Source: CAD feature listing. Evaluate the final solid. Frame: model axes, mm. A direction names the side the tool comes from. Coordinates: 2 decimals unless noted, no trailing zeros. Order: outer loops, then holes, each group sorted by start corner. A loop starts at its lowest first (then second) coordinate and runs counter-clockwise, first axis right, second up. Notation, with made-up numbers: (-12.75, -3.75) -> (27.25, -3.75) arc R29 cw to (27.25, 32.25) -> close; hole circle Ø1 at (83.5, -31). An arc over 180 degrees is marked (long way). Write item = value, one per line. Start each with the question number.
Item 1: Ray query, line 1 along Y through (x, z) = (6, 0.9); line 2 along Y through (x, z) = (-2, 0.3); line 3 along X through (y, z) = (8, 0.9). Return the intervals inside material, ascending. Write a range as [from, to].
Item 2: Section query D-D (x = 8). Output: boundary loops of the cut face in (y, z), then the cut area to 3 significant figures.
Item 3: Contact query for flat-ended pins moving along their axis: pin 1 (0.8 mm diameter, centred on x = 4, z = 0.5, fed in from +Y); pin 2 (0.8 mm diameter, centred on x = -2.5, z = 0.5, fed in from -Y). Output: stop coordinate, or through.
Item 4: Section query B-B (x = -5). Output: boundary loops of the cut face in (y, z).
Item 5: Mould query, pull axis Y, two halves, no side actions, for faces 4 (the flat face through (14, 17, 1)), 5 (the flat face through (0, -11.75, 1)), 6 (the flat face through (-17, -17.75, 1)). Classes: released by +Y, released by -Y, zero draft, split by the parting line, or undercut.
Item 6: Section query A-A (y = 1.25). Output: boundary loops of the cut face in (x, z), then the cut area to 3 significant figures.
Item 7: Section query C-C (z = 0.6). Count the separate pieces of the cut face and the enclosed holes in it, then the cut area to 3 significant figures.
Item 8: Set-up query: faces 1 (the flat face through (17, 17.75, 1)), 2 (the flat face through (0, -13.75, 1)), 3 (the cylindrical face through (-6.53, -4.64, 0.74)). Return all of +Z, -Z, +X, -X, +Y, -Y with unobstructed straight access to the full face (end or side cutting, diameter ignored); none if empty.
```python
from build123d import *

# Parameters (mm, degrees)
F1_DEPTH = 1.5


# Not quite as in the source:
# - ends of sketch curves that miss each other by under 0.0002 mm in the source are joined


with BuildPart() as f1:
    # F0 (on Top) → F1 (new body)
    with BuildSketch(Plane.XY):
        with BuildLine():
            ThreePointArc((19.6082164698, -11.4503983868), (13.339608, 1.2499996959), (19.608215987, 13.9503980169))
            ThreePointArc((19.608215987, 13.9503980169), (19.8967236619, 14.3015730303), (20.000004, 14.744172))
            Line((20.000004, 14.744172), (20.000004, 17.25))
            ThreePointArc((20.000004, 17.25), (19.8535573906, 17.6035533906), (19.500004, 17.75))
            Line((19.500004, 17.75), (14.500004, 17.75))
            ThreePointArc((14.500004, 17.75), (14.1464506094, 17.6035533906), (14.000004, 17.25))
            Line((14.000004, 17.25), (14.000004, 16.25))
            ThreePointArc((14.000004, 16.25), (13.4441182966, 15.5255556337), (12.6004849604, 15.8749999771))
            ThreePointArc((12.6004849604, 15.8749999771), (12.3259659886, 16.1495190594), (11.950966, 16.25))
            Line((11.950966, 16.25), (-11.950958, 16.25))
            ThreePointArc((-11.950958, 16.25), (-12.3259579886, 16.1495190594), (-12.6004770396, 15.8750000229))
            ThreePointArc((-12.6004770396, 15.8750000229), (-13.4441102966, 15.5255556337), (-13.999996, 16.25))
            Line((-13.999996, 16.25), (-13.999996, 17.25))
            ThreePointArc((-13.999996, 17.25), (-14.1464426094, 17.6035533906), (-14.499996, 17.75))
            Line((-14.499996, 17.75), (-19.499996, 17.75))
            ThreePointArc((-19.499996, 17.75), (-19.8535493906, 17.6035533906), (-19.999996, 17.25))
            Line((-19.999996, 17.25), (-19.999996, 14.744172))
            ThreePointArc((-19.999996, 14.744172), (-19.8967156619, 14.3015730303), (-19.6082083041, 13.9503976031))
            ThreePointArc((-19.6082083041, 13.9503976031), (-13.3396, 1.2499996959), (-19.6082084698, -11.4503983868))
            ThreePointArc((-19.6082084698, -11.4503983868), (-19.8967227718, -11.8015703601), (-20.000004, -12.244173))
            Line((-20.000004, -12.244173), (-19.999996, -17.25))
            ThreePointArc((-19.999996, -17.25), (-19.8535493906, -17.6035533906), (-19.499996, -17.75))
            Line((-19.499996, -17.75), (-14.499996, -17.75))
            ThreePointArc((-14.499996, -17.75), (-14.1464426094, -17.6035533906), (-13.999996, -17.25))
            Line((-13.999996, -17.25), (-13.999996, -13.75))
            ThreePointArc((-13.999996, -13.75), (-13.4441102966, -13.0255556337), (-12.6004769604, -13.3749999771))
            ThreePointArc((-12.6004769604, -13.3749999771), (-12.3259579886, -13.6495190594), (-11.950958, -13.75))
            Line((-11.950958, -13.75), (11.950966, -13.75))
            ThreePointArc((11.950966, -13.75), (12.3259659886, -13.6495190594), (12.6004850396, -13.3750000229))
            ThreePointArc((12.6004850396, -13.3750000229), (13.4441182966, -13.0255556337), (14.000004, -13.75))
            Line((14.000004, -13.75), (14.000004, -17.25))
            ThreePointArc((14.000004, -17.25), (14.1464506094, -17.6035533906), (14.500004, -17.75))
            Line((14.500004, -17.75), (19.500004, -17.75))
            ThreePointArc((19.500004, -17.75), (19.8535573906, -17.6035533906), (20.000004, -17.25))
            Line((20.000004, -17.25), (20.000004, -12.244173))
            ThreePointArc((20.000004, -12.244173), (19.8967236619, -11.8015740303), (19.6082164698, -11.4503983868))
        make_face()
        with BuildLine():
            ThreePointArc((-8.6748168, -5.9830934), (-6.4973578405, -4.6318753463), (-3.9800720916, -5.1118651461))
            ThreePointArc((-3.9800720916, -5.1118651461), (3.5765e-06, -6.257042), (3.980079547, -5.1118658719))
            ThreePointArc((3.980079547, -5.1118658719), (6.4973651354, -4.631875401), (8.67482416, -5.98309388))
            Line((8.67482416, -5.98309388), (11.800004, -10.15))
            ThreePointArc((11.800004, -10.15), (11.894431191, -11.1972135955), (11.000004, -11.75))
            Line((11.000004, -11.75), (-10.999996, -11.75))
            ThreePointArc((-10.999996, -11.75), (-11.894423191, -11.1972135955), (-11.799996, -10.15))
            Line((-11.799996, -10.15), (-8.6748168, -5.9830934))
        make_face(mode=Mode.SUBTRACT)
        with BuildLine():
            ThreePointArc((9.000004, 2.95), (10.700004, 1.25), (9.000004, -0.45))
            Line((9.000004, -0.45), (-8.999996, -0.45))
            ThreePointArc((-8.999996, -0.45), (-10.699996, 1.25), (-8.999996, 2.95))
            Line((-8.999996, 2.95), (9.000004, 2.95))
        make_face(mode=Mode.SUBTRACT)
        with BuildLine():
            Line((-10.999996, 14.25), (11.000004, 14.25))
            ThreePointArc((11.000004, 14.25), (11.894431191, 13.6972135955), (11.800004, 12.65))
            Line((11.800004, 12.65), (8.674824, 8.483093))
            ThreePointArc((8.674824, 8.483093), (6.4973648742, 7.1318743525), (3.9800786415, 7.6118644285))
            ThreePointArc((3.9800786415, 7.6118644285), (3.5765e-06, 8.757041), (-3.9800718144, 7.6118647041))
            ThreePointArc((-3.9800718144, 7.6118647041), (-6.4973575792, 7.1318742978), (-8.6748168, 8.4830924))
            Line((-8.6748168, 8.4830924), (-11.799996, 12.65))
            ThreePointArc((-11.799996, 12.65), (-11.894423191, 13.6972135955), (-10.999996, 14.25))
        make_face(mode=Mode.SUBTRACT)
    extrude(amount=F1_DEPTH)


solid = f1.part
```
Computed:
q1.line_1 = [-13.75, -11.75], [-4.58, -0.45], [2.95, 7.08], [14.25, 16.25]
q1.line_2 = [-13.75, -11.75], [-5.99, -0.45], [2.95, 8.49], [14.25, 16.25]
q1.line_3 = [-14.83, -8.24], [-3.28, 3.28], [8.24, 14.83]
q2.outline = (-13.75, 0) -> (-11.75, 0) -> (-11.75, 1.5) -> (-13.75, 1.5) -> close; (-5.3, 0) -> (-0.45, 0) -> (-0.45, 1.5) -> (-5.3, 1.5) -> close; (2.95, 0) -> (7.8, 0) -> (7.8, 1.5) -> (2.95, 1.5) -> close; (14.25, 0) -> (16.25, 0) -> (16.25, 1.5) -> (14.25, 1.5) -> close
q2.area = 20.6 mm^2
q3.pin_1 = 16.25
q3.pin_2 = -13.75
q4.outline = (-13.75, 0) -> (-11.75, 0) -> (-11.75, 1.5) -> (-13.75, 1.5) -> close; (-4.68, 0) -> (-0.45, 0) -> (-0.45, 1.5) -> (-4.68, 1.5) -> close; (2.95, 0) -> (7.18, 0) -> (7.18, 1.5) -> (2.95, 1.5) -> close; (14.25, 0) -> (16.25, 0) -> (16.25, 1.5) -> (14.25, 1.5) -> close
q5.face_4 = zero draft
q5.face_5 = undercut
q5.face_6 = released by -Y
q6.outline = (-13.34, 0) -> (-10.7, 0) -> (-10.7, 1.5) -> (-13.34, 1.5) -> close; (10.7, 0) -> (13.34, 0) -> (13.34, 1.5) -> (10.7, 1.5) -> close
q6.area = 7.92 mm^2
q7.separate_pieces = 1
q7.enclosed_holes = 3
q7.area = 681 mm^2
q8.face_1 = +Z, -Z, +X, -X, +Y
q8.face_2 = +Z, -Z, -Y
q8.face_3 = +Z, -Z
